Input: part model. Units: mm. Frame: model coordinates. Give positions to 0.01 mm unless a question says otherwise; leave off trailing zeros. Loops run counter-clockwise (first coordinate to the right, second up) from the corner with the lowest first, then second, coordinate; pieces in that order, holes last. Notation, with made-up numbers: (52, 31) - (89, 31) arc R16 cw to (89, 36) - close; hole circle Ø3 at (70.25, 34.5). An arc over 180 degrees is marked (long way). One line per question, with ' | ' between items. Start each with the question number.
Autodesk Inventor part; units mm, degrees
ref_plane "YZ Plane" through (0, 0, 0) normal (1, 0, 0) x (0, 1, 0)
ref_plane "XZ Plane" through (0, 0, 0) normal (0, 1, 0) x (-1, 0, 0)
ref_plane "XY Plane" through (0, 0, 0) normal (0, 0, 1) x (1, 0, 0)
sketch "Esboço1" plane through (0, 0, 0) normal (0, 0, 1) x (1, 0, 0)
  line L0 (-121, -21) -> (121, -21)
  line L1 (121, -21) -> (121, 21)
  line L2 (121, 21) -> (-121, 21)
  line L3 (-121, 21) -> (-121, -21)
  line L4 (-121, -21) -> (121, 21) construction
  line L5 (121, -21) -> (-121, 21) construction
  point P0 (0, 0)
  dimension "d0" = 242
  dimension "d1" = 42
extrude "Extrusão1" add sketch "Esboço1" along normal blind 3
sketch "Esboço2" plane through (0, 0, 3) normal (0, 0, 1) x (1, 0, 0)
  line L0 (121, 21) -> (-121, 21)
  line L1 (-121, 21) -> (-79, 21)
  line L2 (-79, 21) -> (-79, -21)
  line L3 (-79, -21) -> (-121, -21)
  line L4 (-121, -21) -> (-121, 21)
  line L5 (-115.5, -15.5) -> (-84.5, -15.5)
  line L6 (-84.5, -15.5) -> (-84.5, 15.5)
  line L7 (-84.5, 15.5) -> (-115.5, 15.5)
  line L8 (-115.5, 15.5) -> (-115.5, -15.5)
  line L9 (-115.5, -15.5) -> (-84.5, 15.5) construction
  line L10 (-84.5, -15.5) -> (-115.5, 15.5) construction
  point P0 (0, 0)
  point P1 (-100, 0)
  point P2 (-100, 21)
  point P3 (-100, 15.5)
  point P4 (-121, 0)
  point P5 (-115.5, 0)
  dimension "d4" = 42
  dimension "d5" = 42
  dimension "d6" = 31
  dimension "d7" = 31
hole "Furo1" at (-115.5, 15.5, 3) at (-84.5, 15.5, 3) at (-84.5, -15.5, 3) at (-115.5, -15.5, 3) direction (0, 0, -1) diameter 3 end through all
hole "Furo2" at (-100, 0, 3) direction (0, 0, -1) diameter 23 end through all
mirror "Espelhamento1" about plane through (0, 0, 0) normal (1, 0, 0) of "Furo1", "Furo2"
sketch "Esboço3" plane through (0, 0, 3) normal (0, 0, 1) x (1, 0, 0)
  circle A0 centre (64, 10.5) radius 1.621
  circle A1 centre (64, -10.5) radius 1.621
  circle A2 centre (-64, 10.5) radius 1.621
  circle A3 centre (-64, -10.5) radius 1.621
  point P0 (0, 0)
hole "Furo3" at (64, -10.5, 3) at (64, 10.5, 3) at (-64, 10.5, 3) at (-64, -10.5, 3) direction (0, 0, -1) diameter 4 end through all
sketch "Esboço4" plane through (0, 0, 3) normal (0, 0, 1) x (1, 0, 0)
  line L0 (121, 21) -> (-121, 21)
  line L1 (-121, 21) -> (-121, -21)
  point P0 (0, 0)
  point P1 (0, 0)
  dimension "d29" = 21
  dimension "d30" = 121
hole "Furo4" at (0, 0, 3) direction (0, 0, -1) diameter 20 end through all
properties part number "chapa lateral"
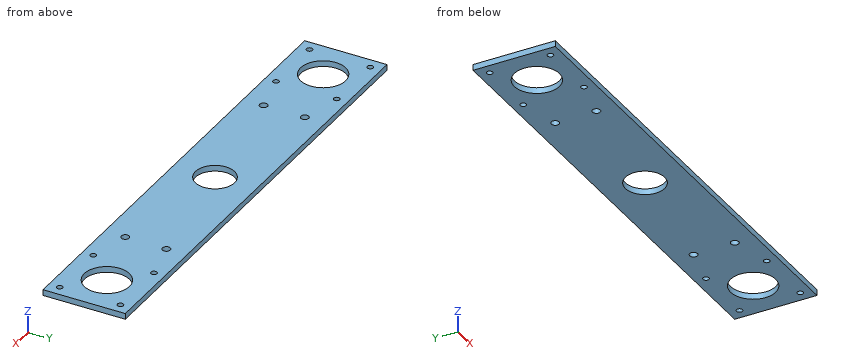
Q1. Section A-A, the plane y = 0. Output: boundary loops of the cut face in (x, z).
Q2. Line query: L1, parallel to Y at x = -115.5, z = 1.7; L2, parallel to X at y = -15.5, z = 0.6; L3, parallel to X at y = 0, z = 1.1. Output: solid intervals per line, ascending. Write a range as from..to.
Q3. Section D-D, the plane x = -96. Output: boundary loops of the cut face in (y, z), plus the area to 3 significant figures.
Q4. Section C-C, the plane x = -64. Output: boundary loops of the cut face in (y, z).
Q5. First-contact query: pin 1 (14 mm diameter, centred on x = -100, y = 0, fed in from +Z). Flat tip, straight axial feed; report the tip coordinate or a pass-through.
Q6. Section B-B, the plane z = 1.35. Count the separate pieces of the cut face and the enclosed holes in it, plus the area to 3 significant figures.
Solved:
1) outline: (-121, 0) - (-111.5, 0) - (-111.5, 3) - (-121, 3) - close; (-88.5, 0) - (-10, 0) - (-10, 3) - (-88.5, 3) - close; (10, 0) - (88.5, 0) - (88.5, 3) - (10, 3) - close; (111.5, 0) - (121, 0) - (121, 3) - (111.5, 3) - close
2) L1: y = -21..-17, -14..14, 17..21 | L2: x = -121..-117, -114..-86, -83..83, 86..114, 117..121 | L3: x = -121..-111.5, -88.5..-10, 10..88.5, 111.5..121
3) outline: (-21, 0) - (-10.78, 0) - (-10.78, 3) - (-21, 3) - close; (10.78, 0) - (21, 0) - (21, 3) - (10.78, 3) - close | area: 61.3 mm²
4) outline: (-21, 0) - (-12.5, 0) - (-12.5, 3) - (-21, 3) - close; (-8.5, 0) - (8.5, 0) - (8.5, 3) - (-8.5, 3) - close; (12.5, 0) - (21, 0) - (21, 3) - (12.5, 3) - close
5) pin 1: passes through
6) separate pieces: 1 | enclosed holes: 15 | area: 8,910 mm²
